Read the model definition and answer for the solid it produces. Units are mm, in the model's axes. Face numbers are marked on the shaded views. Give positions to 0.01 mm unless a question says otherwise; leave off trailing zeros. Order: outer loops, then holes, each group sorted by start corner. A loop starts at its lowest first (then second) coordinate and runs counter-clockwise, first axis right, second up. Notation, with made-up numbers: (37, 37) - (47, 37) arc R10 ccw to (47, 49) - close; hole circle Ø10 at (13.5, 30). An arc over 180 degrees is marked (long way). Write item = value, one per line.
```python
from build123d import *

# Parameters (mm, degrees)
ESQUISSE1_R                 = 122.5
BOSS_EXTRU_1_DEPTH          = 15
ENL_V_MAT_EXTRU_1_OUTLINE_R = 117.5
ENL_V_MAT_EXTRU_1_DEPTH     = 15
ESQUISSE2_R                 = 3.85
ENL_V_MAT_EXTRU_2_DEPTH     = 217.77873659


# Read off the part's stored shape, not the designer's step: Enl_v. mat.-Extru.1
with BuildPart() as part:
    # Esquisse1 → Boss.-Extru.1 (new body)
    with BuildSketch(Plane.XY):
        with Locations((-41.00744319, 19.039170053)):
            Circle(ESQUISSE1_R)
    extrude(amount=BOSS_EXTRU_1_DEPTH)

    # Enl_v. mat.-Extru.1 outline → Enl_v. mat.-Extru.1 (cut)
    with BuildSketch(Plane.XY):
        with Locations((-41.053541595, 19.002849863)):
            Circle(ENL_V_MAT_EXTRU_1_OUTLINE_R)
    extrude(amount=ENL_V_MAT_EXTRU_1_DEPTH, mode=Mode.SUBTRACT)

    # Esquisse2 → Enl_v. mat.-Extru.2 (cut, through all)
    with BuildSketch(Plane(origin=(0, 0, 0), x_dir=(1, 0, 0), z_dir=(0, 1, 0))):
        with Locations(Location((-41.310397507, -7.625301321, 0), (0, 0, 270))):
            Circle(ESQUISSE2_R)
    extrude(amount=-ENL_V_MAT_EXTRU_2_DEPTH, mode=Mode.SUBTRACT)


solid = part.part
```
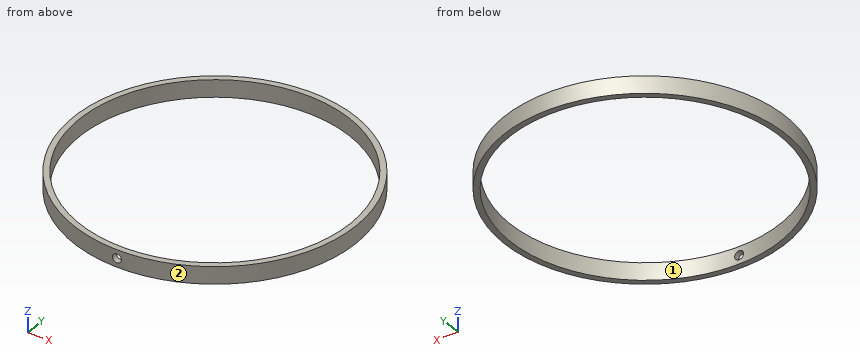
1. Determine the mould class of the marked faces 1 and 2 for opening direction X: +X half, -X half, draft (parallel to the pull), parting line (faces both ways), or undercut.
Recorded:
face_1 = undercut
face_2 = parting line
2. Straight lines are drawn through the part: L1, parallel to Y at x = -100.5, z = 2; L2, parallel to X at y = -36, z = 5; L3, parallel to X at y = -72, z = 10.5 (3 decimals). For each, find the intervals that lie inside material, in ascending order. Write a range as [from, to].
Recorded:
L1 = [-88.04, -82.35], [120.36, 126.12]
L2 = [-150.45, -144.88], [62.78, 68.43]
L3 = [-122.972, -115.382], [33.275, 40.957]
3. Section B-B (y = -31) is taken. Determine the outline of the cut face in (x, z).
Recorded:
outline = (-152.82, 0) - (-147.38, 0) - (-147.38, 15) - (-152.82, 15) - close; (65.28, 0) - (70.81, 0) - (70.81, 15) - (65.28, 15) - close
4. Section A-A (x = -114) is taken. Determine the outline of the cut face in (y, z), and give its area (3 significant figures).
Recorded:
outline = (-79.34, 0) - (-73.11, 0) - (-73.11, 15) - (-79.34, 15) - close; (111.12, 0) - (117.42, 0) - (117.42, 15) - (111.12, 15) - close
area = 188 mm^2
5. Flat-ended cylindrical pins translate along their axes: pin 1 (1 mm diameter, centred on y = 72, z = 5, fed in from -X); pin 2 (2 mm diameter, centred on x = -87.5, z = 5.5, fed in from -Y); pin 3 (2 mm diameter, centred on y = 26.5, z = 6.5, fed in from -X). Find the tip coordinate at first contact, or state that the pin passes through.
Recorded:
pin_1 = -151.71
pin_2 = -94.7
pin_3 = -163.34
6. Section C-C (z = 8) is taken. Determine the outline of the cut face in (x, y).
Recorded:
outline = (-45.14, -103.39) - (-45.14, -98.43) arc R117.5 cw (long way) to (-37.48, -98.44) - (-37.48, -103.41) arc R122.5 ccw (long way) to start
